from build123d import *

# Parameters (mm, degrees)
F1_DEPTH = 25.4
F3_DEPTH = 17.272
F4_W     = 23.310908
F4_H     = 8.280322
F5_DEPTH = 23.876
F7_DEPTH = 50.8


with BuildPart() as f1:
    # F0 (on Front) → F1 (new body)
    with BuildSketch(Plane.XZ):
        with BuildLine():
            Line((23.818642, -36.310196), (23.818642, 44.50167))
            Line((23.818642, 44.50167), (7.39786, 44.50167))
            Line((7.39786, 44.50167), (7.39786, 19.167547))
            ThreePointArc((7.39786, 19.167547), (-0.678108, 10.708378), (-7.09106, 20.488605))
            Line((-7.09106, 20.488605), (-7.09106, 44.50167))
            Line((-7.09106, 44.50167), (-23.818642, 44.50167))
            Line((-23.818642, 44.50167), (-23.818642, -44.50167))
            Line((-23.818642, -44.50167), (16.52839, -44.50167))
            Line((16.52839, -44.50167), (16.52839, -36.310196))
            Line((16.52839, -36.310196), (23.818642, -36.310196))
        make_face()
    extrude(amount=F1_DEPTH)

    # F2 (on Right) → F3 (join)
    with BuildSketch(Plane.YZ):
        Polygon((-25.332414, -44.583075), (-25.396273, -36.345303), (-48.64084, -36.345303), (-48.64084, -44.710793), align=None)
    extrude(amount=F3_DEPTH)

    # F4 (on Right) → F5 (join)
    with BuildSketch(Plane.YZ):
        with Locations((-37.007682, -40.510669)):
            Rectangle(F4_W, F4_H)
    extrude(amount=-F5_DEPTH)

    # F6 (on Front) → F7 (join)
    with BuildSketch(Plane.XZ):
        with BuildLine():
            ThreePointArc((16.882643, -36.605049), (-3.576906, -40.894858), (-23.993824, -36.406536))
            Line((-23.993824, -36.406536), (-23.923699, -40.75424))
            ThreePointArc((-23.923699, -40.75424), (-3.327998, -44.695684), (17.132053, -40.101755))
            Line((17.132053, -40.101755), (17.169088, -36.476661))
            ThreePointArc((17.169088, -36.476661), (17.025967, -36.54108), (16.882643, -36.605049))
        make_face()
        with BuildLine():
            Line((17.239213, -40.052999), (17.169088, -36.476661))
            Line((17.169088, -36.476661), (17.132053, -40.101755))
            ThreePointArc((17.132053, -40.101755), (17.185647, -40.077407), (17.239213, -40.052999))
        make_face()
    extrude(amount=F7_DEPTH)


solid = f1.part
Source: CAD feature listing. Evaluate the final solid. Frame: model axes, mm. A direction names the side the tool comes from. Coordinates: 2 decimals unless noted, no trailing zeros. Order: outer loops, then holes, each group sorted by start corner. A loop starts at its lowest first (then second) coordinate and runs counter-clockwise, first axis right, second up.
Item 1: Cut plane A-A (z = 35). Return loops of the section in (x, y).
Output values:
outline: (-23.82, -25.4) - (-7.09, -25.4) - (-7.09, 0) - (-23.82, 0) - close; (7.4, -25.4) - (23.82, -25.4) - (23.82, 0) - (7.4, 0) - close
Item 2: Pull-direction query (X, two-part tool) for faces 1 (the face through (-0.491, -12.522, 10.694)), 2 (the face through (9, -48.641, -39)), 3 (the face through (-23.819, -12, -43)), 4 (the face through (0, 0, 1)); classes: pulls with the +X half, pulls with the -X half, needs draft (parallel to the pull), parting line crosses it, or undercut.
Output values:
face 1: undercut
face 2: undercut
face 3: pulls with the -X half
face 4: needs draft
Item 3: Cut plane B-B (y = -13.5). Return loops of the section in (x, z).
Output values:
outline: (-23.99, -36.41) - (-23.92, -40.75) arc R51.51 ccw to (-23.82, -40.8) - (-23.82, -44.5) - (-8.69, -44.5) arc R51.51 ccw to (0.39, -44.5) - (16.53, -44.5) - (16.53, -40.37) arc R51.51 ccw to (17.13, -40.1) arc R52.34 ccw to (17.24, -40.05) - (17.17, -36.48) arc R49.9 cw to (16.88, -36.61) arc R49.78 cw to (16.53, -36.76) - (16.53, -36.31) - (23.82, -36.31) - (23.82, 44.5) - (7.4, 44.5) - (7.4, 19.17) arc R7.47 cw (long way) to (-7.09, 20.49) - (-7.09, 44.5) - (-23.82, 44.5) - (-23.82, -36.49) arc R49.78 cw to start
Item 4: Cut plane C-C (x = -10.5). Return loops of the section in (y, z).
Output values:
outline: (-50.8, -44.31) - (-48.66, -44.31) - (-48.66, -44.65) - (-25.35, -44.65) - (-25.35, -44.5) - (0, -44.5) - (0, 44.5) - (-25.4, 44.5) - (-25.4, -36.37) - (-48.66, -36.37) - (-48.66, -40.38) - (-50.8, -40.38) - close
Item 5: Cut plane D-D (z = -28.5). Return loops of the section in (x, y).
Output values:
outline: (-23.82, -25.4) - (23.82, -25.4) - (23.82, 0) - (-23.82, 0) - close
Item 6: First-contact query: P1, Ø17, axis at x = 0, z = 18.15, coming from the -Y side; P2, Ø1.1, axis at y = -18, z = -42.5, coming from the -X side; P3, Ø3, axis at x = -17.5, y = -15, coming from the -Z side. Flat tips, straight axial feed; report the tip coordinate or a pass-through.
Output values:
P1: stops at y = -25.4
P2: stops at x = -23.82
P3: stops at z = -44.5
Item 7: Set-up query: faces 5 (the face through (7.398, -13, 32)), 6 (the face through (0, -25.4, 5)), 7 (the face through (8, -12, -44.502)), 8 (the face through (-19, -48.663, -44)). Return all of +Z, -Z, +X, -X, +Y, -Y with unobstructed straight access to the full face (end or side cutting, diameter ignored); none if empty.
Output values:
face 5: +Z, +Y, -Y
face 6: +Z, +X, -X, -Y
face 7: -Z, +X, +Y
face 8: -Z, -X, -Y
Item 8: Material intervals for line 1 (Z direction, x = 3.5, y = -43.5); line 2 (X direction, y = -8.5, z = -7); line 3 (Y direction, x = 17, z = -10), sorted ascending.
Output values:
line 1: z = -44.68 to -36.35
line 2: x = -23.82 to 23.82
line 3: y = -25.4 to 0
